Geometry check sheet. Reference: the model listing, model coordinates, mm. Face numbers are marked on the shaded views. Give positions to 0.01 mm unless a question says otherwise; leave off trailing zeros. Loops run counter-clockwise (first coordinate to the right, second up) from the corner with the lowest first, then second, coordinate; pieces in that order, holes last. Notation, with made-up numbers: (71.5, 31) -> (101.5, 31) arc R19 ccw to (101.5, 49) -> close; hole circle Ø11 at (-30.5, -12.75). An arc over 180 degrees is marked (long way). Answer in a Markdown table with one row per item. Add a question column.
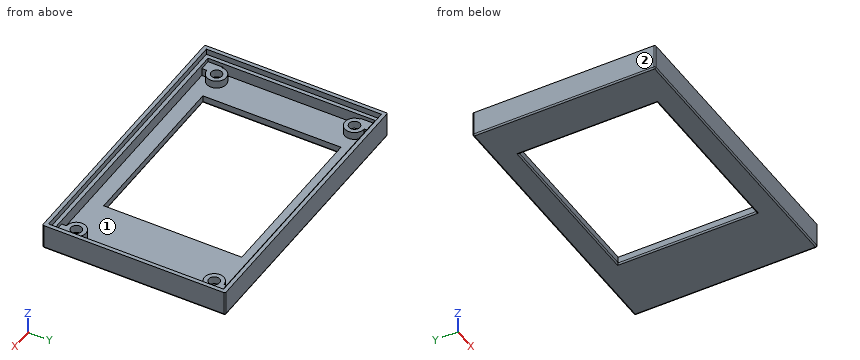
```python
from build123d import *

# Parameters (mm, degrees)
SKETCH1_W           = 72
SKETCH1_H           = 47
BOSS_EXTRUDE1_DEPTH = 6.5
SHELL1_T            = -2
SKETCH2_W           = 44
SKETCH2_H           = 35.5
CUT_EXTRUDE1_DEPTH  = 7.5
SKETCH3_R           = 2.5
BOSS_EXTRUDE2_DEPTH = 2
SKETCH5_W           = 2.75
SKETCH5_H           = 3.79
SKETCH5_H_2         = 3.75
SKETCH5_W_2         = 3.04
BOSS_EXTRUDE3_DEPTH = 2
SKETCH6_R           = 1.4
CUT_EXTRUDE2_DEPTH  = 2
SKETCH7_W           = 70
SKETCH7_H           = 45
CUT_EXTRUDE3_DEPTH  = 1.5
FILLET1_R           = 0.35


with BuildPart() as part:
    # Sketch1 → Boss-Extrude1 (new body)
    with BuildSketch(Plane.XY):
        Rectangle(SKETCH1_W, SKETCH1_H)
    extrude(amount=BOSS_EXTRUDE1_DEPTH)

    # Shell1
    shell1_openings = [part.faces().sort_by_distance(p)[0] for p in [
        (0, 0, 6.5),
    ]]
    offset(amount=SHELL1_T, openings=shell1_openings, kind=Kind.INTERSECTION)

    # Sketch2 → Cut-Extrude1 (cut, through all)
    with BuildSketch(Plane(origin=(0, 0, 0), x_dir=(-1, 0, 0), z_dir=(0, 0, -1))):
        with Locations((3.25, 0)):
            Rectangle(SKETCH2_W, SKETCH2_H)
    extrude(amount=-CUT_EXTRUDE1_DEPTH, mode=Mode.SUBTRACT)

    # Sketch3 → Boss-Extrude2 (add)
    with BuildSketch(Plane.XY.offset(2)):
        with Locations((-31.25, 17.75)):
            Circle(SKETCH3_R)
        with Locations((30.96, 17.75)):
            Circle(SKETCH3_R)
        with Locations((-31.25, -17.71)):
            Circle(SKETCH3_R)
        with Locations((30.96, -17.71)):
            Circle(SKETCH3_R)
    extrude(amount=BOSS_EXTRUDE2_DEPTH)

    # Sketch5 → Boss-Extrude3 (add)
    with BuildSketch(Plane.XY.offset(2)):
        with Locations((-32.625, -19.605)):
            Rectangle(SKETCH5_W, SKETCH5_H)
        with Locations((-32.625, 19.625)):
            Rectangle(SKETCH5_W, SKETCH5_H_2)
        with Locations((32.48, 19.625)):
            Rectangle(SKETCH5_W_2, SKETCH5_H_2)
        with Locations((32.48, -19.605)):
            Rectangle(SKETCH5_W_2, SKETCH5_H)
    extrude(amount=BOSS_EXTRUDE3_DEPTH)

    # Sketch6 → Cut-Extrude2 (cut)
    with BuildSketch(Plane.XY.offset(4)):
        with Locations((-31.25, -17.71)):
            Circle(SKETCH6_R)
        with Locations((-31.25, 17.75)):
            Circle(SKETCH6_R)
        with Locations((30.96, 17.75)):
            Circle(SKETCH6_R)
        with Locations((30.96, -17.71)):
            Circle(SKETCH6_R)
    extrude(amount=-CUT_EXTRUDE2_DEPTH, mode=Mode.SUBTRACT)

    # Sketch7 → Cut-Extrude3 (cut)
    with BuildSketch(Plane.XY.offset(6.5)):
        Rectangle(SKETCH7_W, SKETCH7_H)
    extrude(amount=-CUT_EXTRUDE3_DEPTH, mode=Mode.SUBTRACT)

    # Fillet1
    fillet1_edges = [part.edges().sort_by_distance(p)[0] for p in [
        (18.75, 0, 0),
        (-3.25, -17.75, 0),
        (-25.25, 0, 0),
        (-3.25, 17.75, 0),
        (0, 23.5, 0),
        (36, 0, 0),
        (0, -23.5, 0),
        (-36, 0, 0),
        (-36, 23.5, 3.25),
        (36, 23.5, 3.25),
        (36, -23.5, 3.25),
        (-36, -23.5, 3.25),
    ]]
    fillet(fillet1_edges, radius=FILLET1_R)


solid = part.part
```
1. Sectioned sample at C-C (z = 3). Enter the section's corners in (x, y), plus the area to 3 significant figures.
2. Sectioned sample at D-D (x = 22.5). Enter the section's corners in (y, z), plus the area to 3 significant figures.
3. Sectioned sample at A-A (y = 4.5). Enter the section's corners in (x, z), plus the area to 3 significant figures.
4. Sectioned sample at B-B (x = -12). Enter the section's corners in (y, z).
5. Gauge pin test, flat ends, axial feed: pin 1 Ø3 at (x, y) = (31, 19.5) entering from +Z; pin 2 Ø0.8 at (x, y) = (-31.5, 18) entering from +Z; pin 3 Ø4.5 at (x, y) = (32.5, -19) entering from +Z. Record the tip position at first contact, or that the pin passes through.
6. Release check for a two-part mould opening along Y. For the marked faces 1 and 2 record: released by +Y, released by -Y, zero draft, split by the parting line, or undercut.
7. Material ranges on L1, parallel to X at y = 17, z = 6.25; L2, parallel to Y at x = -1, z = 6; L3, parallel to Y at x = 0.5, z = 4, recorded low to high. Write a range as from..to.
Response:
| question | item | result |
|---|---|---|
| 1 | outline | (-36, -23.15) arc R0.35 ccw to (-35.65, -23.5) -> (35.65, -23.5) arc R0.35 ccw to (36, -23.15) -> (36, 23.15) arc R0.35 ccw to (35.65, 23.5) -> (-35.65, 23.5) arc R0.35 ccw to (-36, 23.15) -> close; hole (-34, -17.71) -> (-33.75, -17.71) arc R2.5 cw (long way) to (-31.25, -20.21) -> (-31.25, -21.5) -> (30.96, -21.5) -> (30.96, -20.21) arc R2.5 cw (long way) to (33.46, -17.71) -> (34, -17.71) -> (34, 17.75) -> (33.46, 17.75) arc R2.5 cw (long way) to (30.96, 20.25) -> (30.96, 21.5) -> (-31.25, 21.5) -> (-31.25, 20.25) arc R2.5 cw (long way) to (-33.75, 17.75) -> (-34, 17.75) -> close; hole circle Ø2.8 at (-31.25, -17.71); hole circle Ø2.8 at (-31.25, 17.75); hole circle Ø2.8 at (30.96, -17.71); hole circle Ø2.8 at (30.96, 17.75) |
| 1 | area | 538 mm2 |
| 2 | outline | (-23.5, 0.35) arc R0.35 ccw to (-23.15, 0) -> (23.15, 0) arc R0.35 ccw to (23.5, 0.35) -> (23.5, 6.5) -> (22.5, 6.5) -> (22.5, 5) -> (21.5, 5) -> (21.5, 2) -> (-21.5, 2) -> (-21.5, 5) -> (-22.5, 5) -> (-22.5, 6.5) -> (-23.5, 6.5) -> close |
| 2 | area | 109 mm2 |
| 3 | outline | (-36, 0.35) arc R0.35 ccw to (-35.65, 0) -> (-25.6, 0) arc R0.35 ccw to (-25.25, 0.35) -> (-25.25, 2) -> (-34, 2) -> (-34, 5) -> (-35, 5) -> (-35, 6.5) -> (-36, 6.5) -> close; (18.75, 0.35) arc R0.35 ccw to (19.1, 0) -> (35.65, 0) arc R0.35 ccw to (36, 0.35) -> (36, 6.5) -> (35, 6.5) -> (35, 5) -> (34, 5) -> (34, 2) -> (18.75, 2) -> close |
| 3 | area | 70.9 mm2 |
| 4 | outline | (-23.5, 0.35) arc R0.35 ccw to (-23.15, 0) -> (-18.1, 0) arc R0.35 ccw to (-17.75, 0.35) -> (-17.75, 2) -> (-21.5, 2) -> (-21.5, 5) -> (-22.5, 5) -> (-22.5, 6.5) -> (-23.5, 6.5) -> close; (17.75, 0.35) arc R0.35 ccw to (18.1, 0) -> (23.15, 0) arc R0.35 ccw to (23.5, 0.35) -> (23.5, 6.5) -> (22.5, 6.5) -> (22.5, 5) -> (21.5, 5) -> (21.5, 2) -> (17.75, 2) -> close |
| 5 | pin 1 | stops at z = 4 |
| 5 | pin 2 | stops at z = 2 |
| 5 | pin 3 | stops at z = 5 |
| 6 | face 1 | undercut |
| 6 | face 2 | zero draft |
| 7 | L1 | x = -36..-35, 35..36 |
| 7 | L2 | y = -23.5..-22.5, 22.5..23.5 |
| 7 | L3 | y = -23.5..-21.5, 21.5..23.5 |
